Build history of the part. All positions in model axes, mm. Give positions to 0.01 mm unless a question says otherwise; leave off trailing zeros. Order: outer loops, then holes, each group sorted by start corner. A loop starts at its lowest first (then second) coordinate and runs counter-clockwise, first axis right, second up. Notation, with made-up numbers: (38, 41.5) -> (53, 41.5) arc R24 ccw to (53, 54.5) -> close; hole circle Ø3 at (30, 88). An arc over 180 degrees is marked (long way). One line per question, with ' | ' between items. Start each with the question number.
(1) Cut at A-A (x = -33). Give the cut face in (y, z), then the cut area to 3 significant figures.
(2) Drill centre lines: L1, parallel to Y at x = 31.5, z = 17; L2, parallel to Y at x = -15.5, z = 12.5; L3, parallel to Y at x = 21, z = 18. Where is each one in solid material? Low to high. Write a range as from..to.
(3) Pull direction Y, two halves, no side cores. Call faces 1 (the face through (-0.595, 29.582, 27.112)), 2 (the face through (-2, 59.333, 16)), 3 (the face through (-2, 16.597, 16)): +Y half, -Y half, draft (parallel to the pull), parting line (faces both ways), or undercut.
from build123d import *

# Parameters (mm, degrees)
F0_W     = 122.3997175694
F0_H     = 42.7361652255
F1_DEPTH = 32.0060774684
F5_D     = 2.54


# Not quite as in the source:
# - the program builds the solid bodies; features that only make, move or delete a surface that nothing else refers to are left out


with BuildPart() as f1:
    # F0 (on Top) → F1 (new body)
    with BuildSketch(Plane.XY):
        with Locations((-1.4522224665, 37.9646681249)):
            Rectangle(F0_W, F0_H)
    extrude(amount=F1_DEPTH)

    # F5 (through all)
    with Locations(Plane(origin=(-62.6520812511, 0, 0), x_dir=(0, -1, 0), z_dir=(-1, 0, 0))):
        with Locations((-28.3709894866, 26.730036363), (-23.6220490187, 17.2120258212), (-28.7239328027, 12.1772345155), (-39.0075407922, 12.403704226), (-39.0968136489, 18.9130250365)):
            Hole(F5_D / 2)


solid = f1.part
Result set:
1) outline: (16.6, 0) -> (59.33, 0) -> (59.33, 32.01) -> (16.6, 32.01) -> close; hole circle Ø2.54 at (23.62, 17.21); hole circle Ø2.54 at (28.37, 26.73); hole circle Ø2.54 at (28.72, 12.18); hole circle Ø2.54 at (39.01, 12.4); hole circle Ø2.54 at (39.1, 18.91) | area: 1,340 mm2
2) L1: y = 16.6..22.37, 24.87..59.33 | L2: y = 16.6..27.5, 29.95..37.74, 40.27..59.33 | L3: y = 16.6..22.63, 24.62..38.21, 39.98..59.33
3) face 1: undercut | face 2: +Y half | face 3: -Y half
